```python
from build123d import *

# Parameters (mm, degrees)
SKETCH_1_R               = 10
SKETCH_1_R_2             = 4
EXTRUDE_1_DEPTH          = 30
SKETCH_2_W               = 10
SKETCH_2_H               = 31
EXTRUDE_2_DEPTH          = 10
SKETCH_3_W               = 10
SKETCH_3_H               = 12
CUT_EXTRUDE_1_DEPTH      = 5
HOLE_WIZARD_3_5_3_5_1_D  = 3.5
PATTERN_CIRCULAR_1_COUNT = 4


with BuildPart() as part:
    # Эскиз1 → Бобышка-Вытянуть1 (new body)
    with BuildSketch(Plane.XY):
        Circle(SKETCH_1_R)
        Circle(SKETCH_1_R_2, mode=Mode.SUBTRACT)
    extrude(amount=EXTRUDE_1_DEPTH)

    # Эскиз2 → Бобышка-Вытянуть2 (add)
    with BuildSketch(Plane(origin=(0, 0, 0), x_dir=(-1, 0, 0), z_dir=(0, 0, -1))):
        with Locations((0, 19.5)):
            Rectangle(SKETCH_2_W, SKETCH_2_H)
    extrude_2 = extrude(amount=-EXTRUDE_2_DEPTH)

    # Эскиз3 → Вырез-Вытянуть1 (cut)
    with BuildSketch(Plane(origin=(0, 0, 0), x_dir=(-1, 0, 0), z_dir=(0, 0, -1))):
        with Locations((0, 29)):
            Rectangle(SKETCH_3_W, SKETCH_3_H)
    cut_extrude_1 = extrude(amount=-CUT_EXTRUDE_1_DEPTH, mode=Mode.SUBTRACT)

    # Диаметр отверстия Ø3.5 (3.5)1 (through all)
    with Locations(Plane(origin=(0, 0, 5), x_dir=(-1, 0, 0), z_dir=(0, 0, -1))):
        with Locations((0, 28)):
            hole_wizard_3_5_3_5_1 = Hole(HOLE_WIZARD_3_5_3_5_1_D / 2)

    # Круговой массив1: Бобышка-Вытянуть2, Вырез-Вытянуть1, Диаметр отверстия Ø3.5 (3.5)1 ×4 about axis
    pattern_circular_1_axis = Axis((0, 0, 0), (0, 0, 1))
    for i in range(1, PATTERN_CIRCULAR_1_COUNT):
        add(extrude_2.rotate(pattern_circular_1_axis, i * 360 / PATTERN_CIRCULAR_1_COUNT))
        add(cut_extrude_1.rotate(pattern_circular_1_axis, i * 360 / PATTERN_CIRCULAR_1_COUNT), mode=Mode.SUBTRACT)
        add(hole_wizard_3_5_3_5_1.rotate(pattern_circular_1_axis, i * 360 / PATTERN_CIRCULAR_1_COUNT), mode=Mode.SUBTRACT)


solid = part.part
```
For this review, take the finished solid that the model builds, in its own axes (mm). A direction names the side the tool comes from. Give positions to 0.01 mm unless a question says otherwise; leave off trailing zeros. Loops run counter-clockwise (first coordinate to the right, second up) from the corner with the lowest first, then second, coordinate; pieces in that order, holes last. Notation, with made-up numbers: M -10,-16 L -5,-16 A20 cw -5,14 Z; hole C 85.5,-10.5 d2. An arc over 180 degrees is marked long. One line per item, written item: value. Start each with the question number.
Q1. Machinability: for faces 1 (the face through (-5, 19, 6)), 2 (the face through (23, 0, 2)), 3 (the face through (0, 30, 5)), which of the approach directions +Z, -Z, +X, -X, +Y, -Y give a long, thin tool a straight path to every point of the face, cutting with its end or side? Answer none if there is none.
Q2. For L1, parallel to Y at x = 0, z = 8.7; L2, parallel to Z at x = -19, y = -3; L3, parallel to Y at x = 21.5, z = 6, list the stretches that pass through material, from the lowest coordinate up.
Q3. Draft analysis for pull direction X (two halves, no side actions). For faces 4 (the face through (26.45, -0.81, 7.53)), 5 (the face through (0, 23, 2)), 6 (the face through (5, 19, 6)), state which applies: released by +X, released by -X, zero draft, split by the parting line, or undercut.
Q4. Add section B-B (z = 4). Give the boundary of the cut face in (x, y).
Q5. Clearance check with flat-ended pins moving along their axes: pin 1 Ø11 at (x, z) = (-26, 2.5) entering from +Y; pin 2 Ø1.5 at (x, z) = (11, 8.5) entering from -Y; pin 3 Ø5 at (x, y) = (-0.5, 32) entering from -Z. State where each tip first meets the part, or that it passes through.
Q6. Add section D-D (y = 28). Give the boundary of the cut face in (x, z).
Q7. Add section A-A (x = 0). Give the boundary of the cut face in (y, z).
Reply:
1. face 1: +Z, -Z, -X, +Y
1. face 2: -Z, +X, +Y, -Y
1. face 3: -Z, +X, -X, +Y
2. L1: -35 to -29.75, -26.25 to -4, 4 to 26.25, 29.75 to 35
2. L2: 0 to 10
2. L3: -5 to 5
3. face 4: undercut
3. face 5: zero draft
3. face 6: released by +X
4. outline: M -23,-5 L -8.66,-5 A10 ccw -5,-8.66 L -5,-23 L 5,-23 L 5,-8.66 A10 ccw 8.66,-5 L 23,-5 L 23,5 L 8.66,5 A10 ccw 5,8.66 L 5,23 L -5,23 L -5,8.66 A10 ccw -8.66,5 L -23,5 Z; hole C 0,0 d8
5. pin 1: y = 5
5. pin 2: y = -5
5. pin 3: z = 5
6. outline: M -5,5 L -1.75,5 L -1.75,10 L -5,10 Z; M 1.75,5 L 5,5 L 5,10 L 1.75,10 Z
7. outline: M -35,5 L -29.75,5 L -29.75,10 L -35,10 Z; M -26.25,5 L -23,5 L -23,0 L -4,0 L -4,30 L -10,30 L -10,10 L -26.25,10 Z; M 4,0 L 23,0 L 23,5 L 26.25,5 L 26.25,10 L 10,10 L 10,30 L 4,30 Z; M 29.75,5 L 35,5 L 35,10 L 29.75,10 Z
